Geometry: see drawing. Coordinates: mm, zero at the bounding-box minimum. A direction names the side the tool comes from. Give positions to 0.01 mm unless a question says otherwise; leave off trailing zeros. Loops run counter-clockwise (first coordinate to the right, second up) from the corner with the lowest first, then second, coordinate; pieces in that order, holes last. Notation, with made-up numbers: (14, -16.75) -> (30, -16.75) arc R17 cw to (30, 4.25) -> close; hole circle Ø2 at (82.25, 42.5). An arc over 180 degrees is marked (long way). Return JSON: item names as keys, results as strings. Group by question number.
(1) Draft query along X for the marked faces 1 and 2. Return one class per face: released by +X, released by -X, zero draft, split by the parting line, or undercut.
(2) Cut plane D-D on y = 26.5. Return loops of the section in (x, z), then the cut area to 4 significant figures.
(3) Cut plane C-C on x = 33.25. Return loops of the section in (y, z).
(4) Cut plane B-B on y = 33.25. Return loops of the section in (x, z).
(5) Cut plane A-A on z = 2.7. Return loops of the section in (x, y), then the cut area to 4 significant figures.
(6) Ray query, line 1 (Y direction, x = 2.75, z = 1.1); line 2 (X direction, y = 25.5, z = 3.6); line 3 (Y direction, x = 29.5, z = 3.55). Return the intervals inside material, ascending. Write a range as from..to.
(7) Pin query (flat end, axial travel): pin 1 (0.9 mm diameter, centred on y = 10, z = 3.5, fed in from -X); pin 2 (10 mm diameter, centred on x = 21, y = 12.5, fed in from +Z); pin 3 (1.4 mm diameter, centred on y = 11.5, z = 2.5, fed in from +X). Return the tip coordinate at first contact, or that it passes through.
(8) Access query for the marked faces 3 and 4. Directions: +Z, -Z, +X, -X, +Y, -Y. A direction counts if a zero-diameter tool reaches every point of the face in a straight line with its end or side. Return the directions, or none.
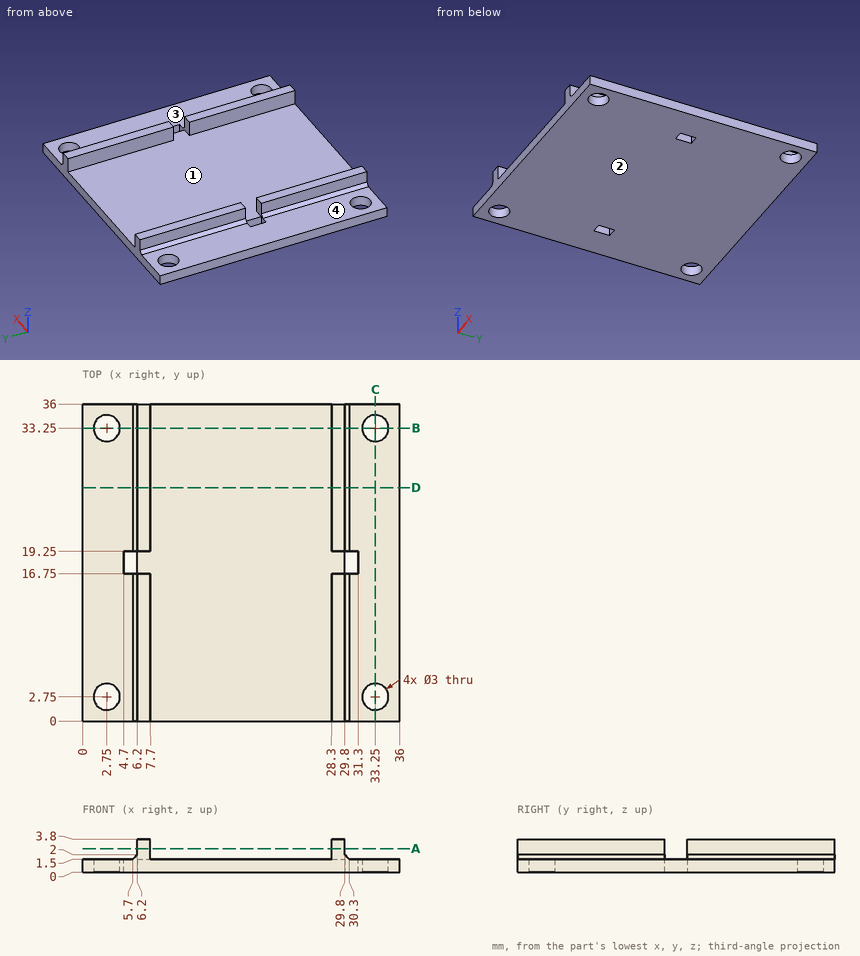
Answers:
{
 "1": {"face 1": "undercut", "face 2": "zero draft"},
 "2": {"outline": "(0, 0) -> (36, 0) -> (36, 1.5) -> (30.3, 1.5) -> (29.8, 2) -> (29.8, 3.8) -> (28.3, 3.8) -> (28.3, 1.5) -> (7.7, 1.5) -> (7.7, 3.8) -> (6.2, 3.8) -> (6.2, 2) -> (5.7, 1.5) -> (0, 1.5) -> close", "area": "61.15 mm²"},
 "3": {"outline": "(0, 0) -> (1.25, 0) -> (1.25, 1.5) -> (0, 1.5) -> close; (4.25, 0) -> (31.75, 0) -> (31.75, 1.5) -> (4.25, 1.5) -> close; (34.75, 0) -> (36, 0) -> (36, 1.5) -> (34.75, 1.5) -> close"},
 "4": {"outline": "(0, 0) -> (1.25, 0) -> (1.25, 1.5) -> (0, 1.5) -> close; (4.25, 0) -> (31.75, 0) -> (31.75, 1.5) -> (30.3, 1.5) -> (29.8, 2) -> (29.8, 3.8) -> (28.3, 3.8) -> (28.3, 1.5) -> (7.7, 1.5) -> (7.7, 3.8) -> (6.2, 3.8) -> (6.2, 2) -> (5.7, 1.5) -> (4.25, 1.5) -> close; (34.75, 0) -> (36, 0) -> (36, 1.5) -> (34.75, 1.5) -> close"},
 "5": {"outline": "(6.2, 0) -> (7.7, 0) -> (7.7, 16.75) -> (6.2, 16.75) -> close; (6.2, 19.25) -> (7.7, 19.25) -> (7.7, 36) -> (6.2, 36) -> close; (28.3, 0) -> (29.8, 0) -> (29.8, 16.75) -> (28.3, 16.75) -> close; (28.3, 19.25) -> (29.8, 19.25) -> (29.8, 36) -> (28.3, 36) -> close", "area": "100.5 mm²"},
 "6": {"line 1": "0..1.25, 4.25..31.75, 34.75..36", "line 2": "6.2..7.7, 28.3..29.8", "line 3": "0..16.75, 19.25..36"},
 "7": {"pin 1": "x = 6.2", "pin 2": "z = 1.5", "pin 3": "x = 30"},
 "8": {"face 3": "+Z, +X, +Y, -Y", "face 4": "+Z, -X, +Y, -Y"}
}
